from build123d import *

# Parameters (mm, degrees)
SKETCH1_R                = 5.0165
SKETCH1_R_2              = 1.778
BOSS_EXTRUDE1_DEPTH      = 9.906
BOSS_EXTRUDE2_DEPTH      = 31.75
BOSS_EXTRUDE2_DEPTH_BACK = 31.75
BOSS_EXTRUDE3_START      = -9.906
SKETCH4_W                = 12.7
SKETCH4_H                = 6.35
BOSS_EXTRUDE3_DEPTH      = 106.934
BOSS_EXTRUDE4_START      = -41.656
SKETCH5_W                = 12.7
SKETCH5_H                = 25.4
BOSS_EXTRUDE4_DEPTH      = 63.5


with BuildPart() as part:
    # Sketch1 → Boss-Extrude1 (new body)
    with BuildSketch(Plane(origin=(0, 0, 0), x_dir=(0, 0, -1), z_dir=(1, 0, 0))):
        with BuildLine():
            Line((-6.35, 10.998522628), (-6.35, 61.798522628))
            Line((-6.35, 61.798522628), (6.35, 61.798522628))
            Line((6.35, 61.798522628), (6.35, 10.998522628))
            ThreePointArc((6.35, 10.998522628), (0, -12.7), (-6.35, 10.998522628))
        make_face()
        Circle(SKETCH1_R, mode=Mode.SUBTRACT)
        with Locations((-8.128, 0)):
            Circle(SKETCH1_R_2, mode=Mode.SUBTRACT)
        with Locations((8.128, 0)):
            Circle(SKETCH1_R_2, mode=Mode.SUBTRACT)
        with Locations((0, -8.128)):
            Circle(SKETCH1_R_2, mode=Mode.SUBTRACT)
        with Locations((0, 8.128)):
            Circle(SKETCH1_R_2, mode=Mode.SUBTRACT)
    extrude(amount=BOSS_EXTRUDE1_DEPTH)

    # Sketch3 → Boss-Extrude2 (add, two sides: drawn at the far end of the back side and taken through both)
    with BuildSketch(Plane(origin=(0, 0, 0), x_dir=(0, 0, -1), z_dir=(1, 0, 0)).offset(-BOSS_EXTRUDE2_DEPTH_BACK)):
        with BuildLine():
            Line((-80.040101608, 104.343522628), (-75.640692557, 106.883522628))
            ThreePointArc((-75.640692557, 106.883522628), (-46.355, 77.597830071), (-6.35, 66.878522628))
            Line((-6.35, 66.878522628), (6.35, 66.878522628))
            ThreePointArc((6.35, 66.878522628), (46.355, 77.597830071), (75.640692557, 106.883522628))
            Line((75.640692557, 106.883522628), (80.040101608, 104.343522628))
            ThreePointArc((80.040101608, 104.343522628), (48.895, 73.19842102), (6.35, 61.798522628))
            Line((6.35, 61.798522628), (-6.35, 61.798522628))
            ThreePointArc((-6.35, 61.798522628), (-48.895, 73.19842102), (-80.040101608, 104.343522628))
        make_face()
    extrude(amount=BOSS_EXTRUDE2_DEPTH + BOSS_EXTRUDE2_DEPTH_BACK)

    # Sketch4 → Boss-Extrude3 (add)
    with BuildSketch(Plane.ZY.offset(BOSS_EXTRUDE3_START)):
        with Locations((0, 33.223522628)):
            Rectangle(SKETCH4_W, SKETCH4_H)
    extrude(amount=-BOSS_EXTRUDE3_DEPTH)

    # Sketch5 → Boss-Extrude4 (add)
    with BuildSketch(Plane(origin=(9.906, 0, 0), x_dir=(0, 0, -1), z_dir=(1, 0, 0)).offset(BOSS_EXTRUDE4_START)):
        with Locations((0, 49.098522628)):
            Rectangle(SKETCH5_W, SKETCH5_H)
    extrude(amount=BOSS_EXTRUDE4_DEPTH)


solid = part.part
Geometry check sheet. Reference: the model listing, model coordinates, mm. A direction names the side the tool comes from. Give positions to 0.01 mm unless a question says otherwise; leave off trailing zeros. Order: outer loops, then holes, each group sorted by start corner. A loop starts at its lowest first (then second) coordinate and runs counter-clockwise, first axis right, second up.
1) Cross-section at C-C (y = 24). Record the boundary of the cut face in (x, z).
Results are:
outline: (0, -6.35) - (9.91, -6.35) - (9.91, 6.35) - (0, 6.35) - close
2) Tool access check on faces 1 (the flat face through (9.906, 9, -3)), 2 (the flat face through (25, 42, -6.35)), 3 (the cylindrical face through (-0.44, 77.89, 46.86)), 4 (the flat face through (31.75, 66.6, 0.4)), 5 (the flat face through (-16, 36.399, 0)). Record the directions out of +Z, -Z, +X, -X, +Y, -Y that give a thin tool (end or side, any length) a straight path to the whole face; none if there is none.
Results are:
face 1: +Z, -Z, +X, -Y
face 2: -Z, +X, -X
face 3: +X, -X, +Y
face 4: +Z, -Z, +X, +Y
face 5: +Z, -Z, -X, -Y
3) Material ranges on probe 1 along Y at (x, z) = (3, 0); probe 2 along X at (y, z) = (22, -5.5); probe 3 along Z at (x, y) = (6.5, 61), recorded low to high.
Results are:
probe 1: y = -12.7 to -9.91, -6.35 to -5.02, 5.02 to 6.35, 9.91 to 66.88
probe 2: x = 0 to 9.91
probe 3: z = -6.35 to 6.35
4) Draft check along Y on faces 6 (the flat face through (25, 42, 6.35)), 7 (the flat face through (-0.444, 105.596, 77.871)), 8 (the flat face through (116.84, 33, 0)). Enter one of: released by +Y, released by -Y, zero draft, split by the parting line, or undercut.
Results are:
face 6: undercut
face 7: released by +Y
face 8: zero draft
5) Gauge pin test, flat ends, axial feed: pin 1 (12 mm diameter, centred on x = -15, z = 15, fed in from +Y); pin 2 (6.5 mm diameter, centred on x = -11.5, z = 3, fed in from -Y); pin 3 (12.5 mm diameter, centred on y = 9, z = 0, fed in from +X). Record the tip position at first contact, or that the pin passes through.
Results are:
pin 1: stops at y = 68.23
pin 2: stops at y = 36.4
pin 3: stops at x = 9.91
6) Cross-section at D-D (z = 67.5). Record the boundary of the cut face in (x, y), then the cut area to 3 significant figures.
Results are:
outline: (-31.75, 87.72) - (31.75, 87.72) - (31.75, 95.29) - (-31.75, 95.29) - close
area: 481 mm2
7) Cross-section at B-B (y = 92). Record the boundary of the cut face in (x, z), then the cut area to 3 significant figures.
Results are:
outline: (-31.75, -71.37) - (31.75, -71.37) - (31.75, -64.56) - (-31.75, -64.56) - close; (-31.75, 64.56) - (31.75, 64.56) - (31.75, 71.37) - (-31.75, 71.37) - close
area: 864 mm2
8) Cross-section at A-A (x = -2). Record the boundary of the cut face in (y, z).
Results are:
outline: (36.4, -6.35) - (61.8, -6.35) arc R85.09 ccw to (104.34, -80.04) - (106.88, -75.64) arc R80.01 cw to (66.88, -6.35) - (66.88, 6.35) arc R80.01 cw to (106.88, 75.64) - (104.34, 80.04) arc R85.09 ccw to (61.8, 6.35) - (36.4, 6.35) - close
